from build123d import *

# Parameters (mm, degrees)
BOSS_EXTRUDE1_DEPTH = 60
BOSS_EXTRUDE2_DEPTH = 60
SKETCH4_W           = 60
SKETCH4_H           = 14.412520708
CUT_EXTRUDE1_DEPTH  = 60


with BuildPart() as part:
    # Sketch2 → Boss-Extrude1 (new body)
    with BuildSketch(Plane.XY):
        Polygon((7.8, 0), (5.515432893, 5.515432893), (0, 7.8), (-5.515432893, 5.515432893), (-7.8, 0), (-5.515432893, -5.515432893), (0, -7.8), (5.515432893, -5.515432893), align=None)
    extrude(amount=BOSS_EXTRUDE1_DEPTH)

    # Sketch3 → Boss-Extrude2 (add)
    with BuildSketch(Plane.XY.offset(60)):
        with BuildLine():
            ThreePointArc((-5.515432893, 5.515432893), (-2.284567107, 5.515432893), (0, 7.8))
            ThreePointArc((0, 7.8), (2.284567107, 5.515432893), (5.515432893, 5.515432893))
            ThreePointArc((5.515432893, 5.515432893), (5.515432893, 2.284567107), (7.8, 0))
            ThreePointArc((7.8, 0), (5.515432893, -2.284567107), (5.515432893, -5.515432893))
            ThreePointArc((5.515432893, -5.515432893), (2.284567107, -5.515432893), (0, -7.8))
            ThreePointArc((0, -7.8), (-2.284567107, -5.515432893), (-5.515432893, -5.515432893))
            ThreePointArc((-5.515432893, -5.515432893), (-4.916369213, -2.036426805), (-7.8, 0))
            ThreePointArc((-7.8, 0), (-5.515432893, 2.284567107), (-5.515432893, 5.515432893))
        make_face()
    extrude(amount=BOSS_EXTRUDE2_DEPTH)

    # Sketch4 → Cut-Extrude1 (cut)
    with BuildSketch(Plane(origin=(-6.657716447, -2.757716447, 0), x_dir=(0, 0, 1), z_dir=(-0.9238795325112824, -0.3826834323651004, 0))):
        with Locations((90, 0)):
            Rectangle(SKETCH4_W, SKETCH4_H)
    extrude(amount=-CUT_EXTRUDE1_DEPTH, mode=Mode.SUBTRACT)


solid = part.part
Could you check a few things on this model? Use its own coordinates, in mm. Coordinates: 2 decimals unless noted, no trailing zeros. Loops run counter-clockwise (first coordinate to the right, second up) from the corner with the lowest first, then second, coordinate; pieces in that order, holes last.
1. Imagine slicing it at B-B (y = -1). Please give me the cut outline in (x, z).
2. I need wall thicknesses on L1, parallel to X at y = -5.5, z = 49.5; L2, parallel to Y at x = -5.75, z = 50; L3, parallel to Y at x = 2, z = 50. Which ranges of each line are inside material? Lowest first, please.
3. For P1, Ø4, axis at y = 5.5, z = 8, coming from the -X side; P2, Ø1.5, axis at x = -3.5, z = 30.5, coming from the -Y side; P3, Ø1, axis at x = 3.5, z = 42.5, coming from the -Y side, each with a flat end and sliding along its axis, tell me the tip position at first contact or that it passes through.
4. Imagine slicing it at A-A (z = 55.5). Please give me the cut outline in (x, y), and give its area (3 significant figures).
5. Imagine slicing it at C-C (x = 6.25). Please give me the cut outline in (y, z).
Computed values:
1. outline: (-7.39, 0) - (7.39, 0) - (7.39, 60) - (-7.39, 60) - close
2. L1: x = -5.52 to 5.52
2. L2: y = -4.95 to 4.95
2. L3: y = -6.97 to 6.97
3. P1: stops at x = -6.35
3. P2: stops at y = -6.66
3. P3: stops at y = -6.56
4. outline: (-7.8, 0) - (-5.52, -5.52) - (0, -7.8) - (5.52, -5.52) - (7.8, 0) - (5.52, 5.52) - (0, 7.8) - (-5.52, 5.52) - close
4. area: 172 mm2
5. outline: (-3.74, 0) - (3.74, 0) - (3.74, 60) - (-3.74, 60) - close
